```python
from build123d import *

# Parameters (mm, degrees)
F1_DEPTH = 19.05
F2_R     = 2.54
F3_DEPTH = 12.7
F4_R     = 5.08


with BuildPart() as f1:
    # F0 (on Front) → F1 (new body, symmetric)
    with BuildSketch(Plane.XZ):
        with BuildLine():
            Line((-24.119121, -47.33848), (24.140879, -47.327388))
            ThreePointArc((24.140879, -47.327388), (-0.012211, 53.128745), (-24.119121, -47.33848))
        make_face()
    extrude(amount=F1_DEPTH, both=True)

    # F2
    f2_edges = [f1.edges().sort_by_distance(p)[0] for p in [
        (-0.012211, -19.05, 53.128745),
        (-0.012211, 19.05, 53.128745),
    ]]
    fillet(f2_edges, radius=F2_R)

    # F0 (on Front) → F3 (join, symmetric)
    with BuildSketch(Plane.XZ):
        with BuildLine():
            Line((24.140879, -148.927388), (24.140879, -47.327388))
            Line((24.140879, -47.327388), (-24.119121, -47.33848))
            Line((-24.119121, -47.33848), (-24.119121, -148.927388))
            ThreePointArc((-24.119121, -148.927388), (0.010879, -173.057388), (24.140879, -148.927388))
        make_face()
    extrude(amount=F3_DEPTH, both=True)

    # F4
    f4_edges = [f1.edges().sort_by_distance(p)[0] for p in [
        (-24.119121, 12.7, -98.132934),
        (-24.119121, -12.7, -98.132934),
        (24.140879, -12.7, -98.127388),
        (24.140879, 12.7, -98.127388),
    ]]
    fillet(f4_edges, radius=F4_R)


solid = f1.part
```
Can you work these out from the model? Positions are in its coordinate system, mm. A direction names the side the tool comes from. Give positions to 0.01 mm unless a question says otherwise; leave off trailing zeros. Order: outer loops, then holes, each group sorted by start corner. A loop starts at its lowest first (then second) coordinate and runs counter-clockwise, first axis right, second up. Notation, with made-up numbers: M 24.5,-1 L 28.5,-1 A12 ccw 28.5,17 Z; hole C -17.5,23.5 d11. An arc over 180 degrees is marked long. Write item = value, one per line. Start each with the question number.
Q1. I need wall thicknesses on probe 1 along X at (y, z) = (-0.5, -113); probe 2 along Y at (x, z) = (-11, -53.5); probe 3 along X at (y, z) = (11, -0.5). Which ranges of each line are inside material? Lowest first, please. Write a range as [from, to].
Q2. Will these pins go through, and if not, where does the flat tip stop? pin 1 Ø2 at (y, z) = (-13, 24.5) entering from -X; pin 2 Ø2 at (x, z) = (-7, -51) entering from +Y; pin 3 Ø5.5 at (x, y) = (-1.5, -13) entering from -Z.
Q3. For faces 1 (the flat face through (-24.119, 0, -97)), 2 (the flat face through (0, -12.7, -107)), 3 (the flat face through (24.141, 0, -99)), which set-ups out of +Z, -Z, +X, -X, +Y, -Y let a thin tool reach every point of the face, with its end or its side?
Q4. Suppose I cut it at A-A (z = -124). Write out the boundary of the cut face in (x, y).
Q5. Suppose I cut it at C-C (y = -10). Write out the boundary of the cut face in (x, z), plus the area to 3 significant figures.
Q6. Suppose I cut it at B-B (y = 3.5). Write out the boundary of the cut face in (x, z), plus the area to 3 significant figures.
Check result:
q1.probe_1 = [-24.12, 24.14]
q1.probe_2 = [-12.7, 12.7]
q1.probe_3 = [-53.13, 53.13]
q2.pin_1 = -47.65
q2.pin_2 = 12.7
q2.pin_3 = -172.28
q3.face_1 = -Z, -X, +Y, -Y
q3.face_2 = -Z, +X, -X, -Y
q3.face_3 = -Z, +X, +Y, -Y
q4.outline = M -24.12,-7.62 A5.08 ccw -19.04,-12.7 L 19.06,-12.7 A5.08 ccw 24.14,-7.62 L 24.14,7.62 A5.08 ccw 19.06,12.7 L -19.04,12.7 A5.08 ccw -24.12,7.62 Z
q5.outline = M -24.12,-47.34 L -23.53,-47.34 L -23.53,-148.93 A23.54 ccw 23.55,-148.93 L 23.55,-47.33 L 24.14,-47.33 A53.13 ccw long Z
q5.area = 14,300 mm2
q6.outline = M -24.12,-148.93 A24.13 ccw 24.14,-148.93 L 24.14,-47.33 A53.13 ccw long -24.12,-47.34 Z
q6.area = 14,500 mm2
